Check sheet for the modelled part. Datum: model origin and axes. Units: mm. A direction names the side the tool comes from. Round coordinates to 2 decimals unless told otherwise and drop trailing zeros. Write each loop counter-clockwise with the first axis right and the second up, starting at its lowest first coordinate (ties: lowest second). Pieces come first, ordered by that corner, then holes. Notation, with made-up numbers: (88, 54.5) -> (109, 54.5) arc R15 ccw to (109, 77.5) -> close; hole circle Ø6 at (-1, 23). An arc over 180 degrees is marked (long way). One line per item, written item: value.
Autodesk Inventor part; units mm, degrees
ref_plane "YZ Plane" through (0, 0, 0) normal (1, 0, 0) x (0, 1, 0)
ref_plane "XZ Plane" through (0, 0, 0) normal (0, 1, 0) x (-1, 0, 0)
ref_plane "XY Plane" through (0, 0, 0) normal (0, 0, 1) x (1, 0, 0)
sketch "Sketch1" plane through (0, 0, 0) normal (0, 0, 1) x (1, 0, 0)
  circle A0 centre (0, 0) radius 7.5
  circle A1 centre (0, 0) radius 10
  dimension "d0" = 15
  dimension "d1" = 20
extrude "Extrusion1" add sketch "Sketch1" along normal blind 1
sketch "Sketch2" plane through (0, 0, 1) normal (0, 0, 1) x (1, 0, 0)
  circle A0 centre (0, 0) radius 8.5
  circle A1 centre (0, 0) radius 7.5
  dimension "d4" = 17
extrude "Extrusion2" add sketch "Sketch2" along normal blind 6
chamfer "Chamfer1" distance 0.5 angle 45 1 edges at (-8.5, 0, 7)
properties part number "オイレス" material "Acetal Resin, Black"
Item 1: Mould release check, pull along X, two halves, no side actions. Record for faces 3 (the cylindrical face through (-7.493, -0.33, 3.451)), 4 (the cylindrical face through (4.57, -7.167, 3.712)), 5 (the flat face through (4, 7, 0)): pulls with the +X half, pulls with the -X half, needs draft (parallel to the pull), parting line crosses it, or undercut.
Answer:
face 3: undercut
face 4: parting line crosses it
face 5: needs draft
Item 2: Sectioned sample at C-C on z = 2.75. Enter the section's corners in (x, y).
Answer:
outline: circle Ø17 at (0, 0); hole circle Ø15 at (0, 0)
Item 3: Thickness scan on line 1 (Y direction, x = 0, z = 5.25); line 2 (Z direction, x = -3.25, y = -9); line 3 (Y direction, x = 5.25, z = 1.75). Record the ranges inside material, lowest first.
Answer:
line 1: y = -8.5 to -7.5, 7.5 to 8.5
line 2: z = 0 to 1
line 3: y = -6.68 to -5.36, 5.36 to 6.68
Item 4: Sectioned sample at A-A on y = 0. Enter the section's corners in (x, z).
Answer:
outline: (-10, 0) -> (-7.5, 0) -> (-7.5, 7) -> (-8, 7) -> (-8.5, 6.5) -> (-8.5, 1) -> (-10, 1) -> close; (7.5, 0) -> (10, 0) -> (10, 1) -> (8.5, 1) -> (8.5, 6.5) -> (8, 7) -> (7.5, 7) -> close
Item 5: Depth check by flat-ended pin: P1, Ø2, axis at x = -1, z = 3, coming from the +Y side; P2, Ø1.5, axis at y = 3.5, z = 2.5, coming from the +X side; P3, Ø2, axis at y = -3, z = 3, coming from the +X side. Enter the tip coordinate at first touch or a pass-through.
Answer:
P1: stops at y = 8.5
P2: stops at x = 8.04
P3: stops at x = 8.26
Item 6: Tool access check on faces 1 (the cylindrical face through (-2.17, 9.76, 0.49)), 2 (the flat face through (-4.5, -7.4, 1)). Record the directions out of +Z, -Z, +X, -X, +Y, -Y that give a thin tool (end or side, any length) a straight path to the whole face; none if there is none.
Answer:
face 1: +Z, -Z
face 2: +Z
